Could you check a few things on this drawing? It's one solid part, dimensions in mm from its lowest x, y, z. Round coordinates to 2 decimals unless told otherwise and drop trailing zeros. Order: outer loops, then holes, each group sorted by start corner. A loop starts at its lowest first (then second) coordinate and runs counter-clockwise, first axis right, second up.
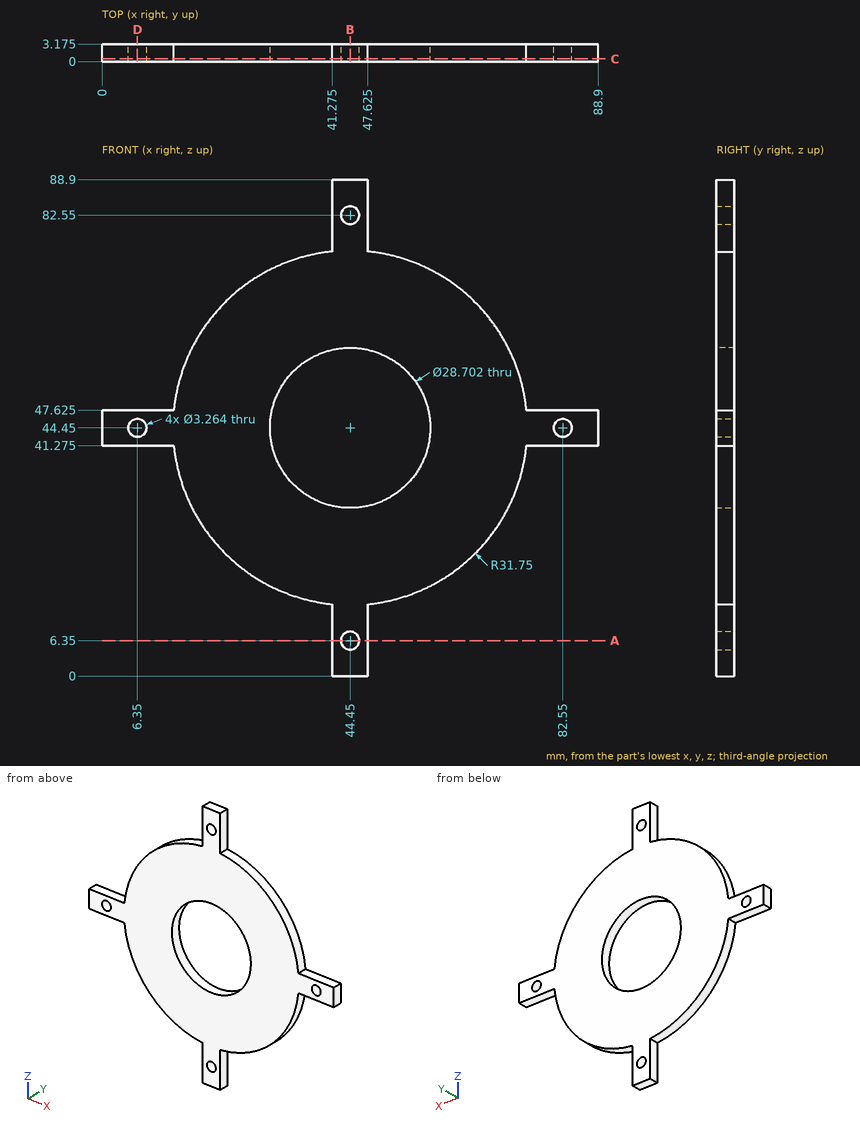
(1) I want a section at D-D, the plane x = 6.35. List the corners of the cut face in (y, z) for me (3 decimals).
(2) I want a section at B-B, the plane x = 44.45. List the corners of the cut face in (y, z) for me (3 decimals).
(3) I'm going to push flat-ended pins straight in: pin 1 Ø1.6 at (x, y) = (82.5, 1.5) entering from -Z (3 decimals); pin 2 Ø1 at (x, y) = (85, 1.5) entering from +Z (3 decimals); pin 3 Ø1 at (x, y) = (15, 2) entering from -Z. Where does each tip first touch, or does it pass through?
(4) I want a section at C-C, the plane y = 0.5. List the corners of the cut face in (x, z) for me (3 decimals), plus the area to 3 significant figures.
(5) I want a section at A-A, the plane z = 6.35. List the corners of the cut face in (x, y) for me (3 decimals).
(6) Please list where these lines run through material, in increasing order: probe 1 along Z at (x, y) = (6.35, 2.5) (3 decimals); probe 2 along Z at (x, y) = (44, 0.4); probe 3 along X at (y, z) = (1.25, 10) (3 decimals).
Ans:
1. outline: (0, 41.275) - (3.175, 41.275) - (3.175, 42.818) - (0, 42.818) - close; (0, 46.082) - (3.175, 46.082) - (3.175, 47.625) - (0, 47.625) - close
2. outline: (0, 0) - (3.175, 0) - (3.175, 4.718) - (0, 4.718) - close; (0, 7.982) - (3.175, 7.982) - (3.175, 30.099) - (0, 30.099) - close; (0, 58.801) - (3.175, 58.801) - (3.175, 80.918) - (0, 80.918) - close; (0, 84.182) - (3.175, 84.182) - (3.175, 88.9) - (0, 88.9) - close
3. pin 1: stops at z = 41.275
3. pin 2: stops at z = 47.625
3. pin 3: stops at z = 31.41
4. outline: (0, 41.275) - (12.859, 41.275) arc R31.75 ccw to (41.275, 12.859) - (41.275, 0) - (47.625, 0) - (47.625, 12.859) arc R31.75 ccw to (76.041, 41.275) - (88.9, 41.275) - (88.9, 47.625) - (76.041, 47.625) arc R31.75 ccw to (47.625, 76.041) - (47.625, 88.9) - (41.275, 88.9) - (41.275, 76.041) arc R31.75 ccw to (12.859, 47.625) - (0, 47.625) - close; hole circle Ø3.264 at (6.35, 44.45); hole circle Ø28.702 at (44.45, 44.45); hole circle Ø3.264 at (44.45, 6.35); hole circle Ø3.264 at (44.45, 82.55); hole circle Ø3.264 at (82.55, 44.45)
4. area: 2,810 mm2
5. outline: (41.275, 0) - (42.818, 0) - (42.818, 3.175) - (41.275, 3.175) - close; (46.082, 0) - (47.625, 0) - (47.625, 3.175) - (46.082, 3.175) - close
6. probe 1: z = 41.275 to 42.818, 46.082 to 47.625
6. probe 2: z = 0 to 4.78, 7.92 to 30.11, 58.79 to 80.98, 84.12 to 88.9
6. probe 3: x = 41.275 to 47.625
